```python
from build123d import *

# Parameters (mm, degrees)
SKETCH1_W           = 249.00380235
SKETCH1_H           = 131.677440474
BOSS_EXTRUDE1_DEPTH = 192
CHAMFER1_SIZE       = 100
SKETCH2_W           = 249.00380235
SKETCH2_H           = 141.421356237
SKETCH2_W_2         = 215.26057226
SKETCH2_H_2         = 100.329330499
BOSS_EXTRUDE2_DEPTH = 10
SHELL1_START        = -114.501901175
SHELL1_DEPTH        = 229.00380235
BOSS_EXTRUDE3_DEPTH = 5
SKETCH4_W           = 5
SKETCH4_H           = 182
BOSS_EXTRUDE4_DEPTH = 5


# Read off the part's stored shape, not the designer's step: Shell1
with BuildPart() as part:
    # Sketch1 → Boss-Extrude1 (new body)
    with BuildSketch(Plane(origin=(0, 0, 0), x_dir=(1, 0, 0), z_dir=(0, 1, 0))):
        Rectangle(SKETCH1_W, SKETCH1_H)
    extrude(amount=BOSS_EXTRUDE1_DEPTH)

    # Chamfer1
    chamfer1_edges = [part.edges().sort_by_distance(p)[0] for p in [
        (0, 192, 65.838720237),
    ]]
    chamfer(chamfer1_edges, length=CHAMFER1_SIZE)

    # Sketch2 → Boss-Extrude2 (add)
    with BuildSketch(Plane(origin=(0, 78.919360119, 78.919360119), x_dir=(1, 0, 0), z_dir=(0, 0.7071067811865464, 0.7071067811865487))):
        with Locations((0, 89.209496444)):
            Rectangle(SKETCH2_W, SKETCH2_H)
        with Locations((0, 89.209496444)):
            Rectangle(SKETCH2_W_2, SKETCH2_H_2, mode=Mode.SUBTRACT)
    extrude(amount=BOSS_EXTRUDE2_DEPTH)

    # Shell1 outline → Shell1 (cut)
    with BuildSketch(Plane.YZ.offset(SHELL1_START)):
        Polygon((96.142135624, 55.838720237), (10, 55.838720237), (10, -65.838720237), (182, -65.838720237), (182, -30.019144139), (184.928932188, -27.090211951), (99.071067812, 58.767652425), align=None)
    extrude(amount=SHELL1_DEPTH, mode=Mode.SUBTRACT)

    # Sketch3 → Boss-Extrude3 (add)
    with BuildSketch(Plane(origin=(0, 0, -65.838720237), x_dir=(-1, 0, 0), z_dir=(0, 0, -1))):
        Polygon((-114.501901175, 10), (-114.501901175, 182), (-114.501901175, 192), (-124.501901175, 192), (-124.501901175, 0), (124.501901175, 0), (124.501901175, 192), (114.501901175, 192), (114.501901175, 182), (114.501901175, 10), align=None)
    extrude(amount=BOSS_EXTRUDE3_DEPTH)

    # Sketch4 → Boss-Extrude4 (add)
    with BuildSketch(Plane(origin=(0, 0, -70.838720237), x_dir=(-1, 0, 0), z_dir=(0, 0, -1))):
        Polygon((124.501901175, 192), (114.501901175, 192), (114.501901175, 10), (-114.501901175, 10), (-114.501901175, 192), (-124.501901175, 192), (-124.501901175, 0), (124.501901175, 0), align=None)
        with Locations((112.001901175, 101)):
            Rectangle(SKETCH4_W, SKETCH4_H)
        with Locations((-112.001901175, 101)):
            Rectangle(SKETCH4_W, SKETCH4_H)
    extrude(amount=BOSS_EXTRUDE4_DEPTH)


solid = part.part
```
Geometry: final body of the model. Coordinates: model frame, mm. A direction names the side the tool comes from. Round coordinates to 2 decimals unless told otherwise and drop trailing zeros. Write each loop counter-clockwise with the first axis right and the second up, starting at its lowest first coordinate (ties: lowest second). Pieces come first, ordered by that corner, then holes. Notation, with made-up numbers: (66.5, -17.75) -> (91.5, -17.75) arc R24 ccw to (91.5, 6.25) -> close; hole circle Ø8 at (45.5, 6.25). An arc over 180 degrees is marked (long way). Use CSV: the item, a comma, the result in double quotes. Start each with the question number.
Q1. Section D-D (z = 23). Return loops of the section in (x, y), plus the area to 3 significant figures.
Q2. Line query: L1, parallel to Y at x = -92, z = -65; L2, parallel to X at y = 25.5, z = -51; L3, parallel to Z at x = -114, y = 91. Output: solid intervals per line, ascending.
Q3. Section B-B (x = 27). Return loops of the section in (y, z).
Q4. First-contact query: pin 1 Ø2.5 at (x, y) = (-112, 128) entering from +Z; pin 2 Ø8 at (x, z) = (13, -18) entering from +Y; pin 3 Ø5.5 at (x, y) = (111, 82) entering from +Z; pin 4 Ø18 at (x, z) = (25.5, -43) entering from -Y. Flat tips, straight axial feed; report the tip coordinate or a pass-through.
Q5. Section A-A (y = 15). Return loops of the section in (x, z).
Q6. Section C-C (y = 160). Return loops of the section in (x, z), plus the area to 3 significant figures.
Q7. Reachability of faces 5 (the face through (-2, 192, -50)), 6 (the face through (-114.502, 82, -5)), 7 (the face through (-1.507, 110.014, 54.797)), 8 (the face through (-1.743, 95.486, 69.325)), 9 (the face through (-1.507, 180.958, -16.147)) from +Z, -Z, +X, -X, +Y, -Y: full face, straight path, thin tool, end or side. Return the list, or none.
Q8. Pull-direction query (X, two-part tool) for faces 1 (the face through (-2, 54, 55.839)), 2 (the face through (-124.502, 76, 0)), 3 (the face through (124.502, 79, -17)), 4 (the face through (-2, 45, 65.839)); classes: pulls with the +X half, pulls with the -X half, needs draft (parallel to the pull), parting line crosses it, or undercut.
Result sheet:
1,outline,"(-124.5, 0) -> (124.5, 0) -> (124.5, 148.98) -> (107.63, 148.98) -> (107.63, 134.84) -> (114.5, 134.84) -> (114.5, 10) -> (-114.5, 10) -> (-114.5, 134.84) -> (-107.63, 134.84) -> (-107.63, 148.98) -> (-124.5, 148.98) -> close"
1,area,"5,460 mm²"
2,L1,"0 to 10, 182 to 192"
2,L2,"-124.5 to -114.5, 114.5 to 124.5"
2,L3,"-75.84 to -70.84, 55.84 to 65.84"
3,outline,"(0, -75.84) -> (10, -75.84) -> (10, 55.84) -> (96.14, 55.84) -> (99.07, 58.77) -> (106.53, 51.31) -> (113.6, 58.38) -> (99.07, 72.91) -> (92, 65.84) -> (0, 65.84) -> close; (177.47, -19.63) -> (184.93, -27.09) -> (182, -30.02) -> (182, -65.84) -> (192, -65.84) -> (192, -34.16) -> (199.07, -27.09) -> (184.54, -12.56) -> close"
4,pin 1,"z = 45.23"
4,pin 2,"y = 193.98"
4,pin 3,"z = 65.84"
4,pin 4,"y = 0"
5,outline,"(-124.5, -75.84) -> (-109.5, -75.84) -> (-109.5, -70.84) -> (-114.5, -70.84) -> (-114.5, 55.84) -> (114.5, 55.84) -> (114.5, -70.84) -> (109.5, -70.84) -> (109.5, -75.84) -> (124.5, -75.84) -> (124.5, 65.84) -> (-124.5, 65.84) -> close"
6,outline,"(-124.5, -75.84) -> (-109.5, -75.84) -> (-109.5, -70.84) -> (-114.5, -70.84) -> (-114.5, -2.16) -> (-107.63, -2.16) -> (-107.63, 11.98) -> (-124.5, 11.98) -> close; (107.63, -2.16) -> (114.5, -2.16) -> (114.5, -70.84) -> (109.5, -70.84) -> (109.5, -75.84) -> (124.5, -75.84) -> (124.5, 11.98) -> (107.63, 11.98) -> close"
6,area,"2,000 mm²"
7,face 5,"-Z, +X, -X, +Y"
7,face 6,"none"
7,face 7,"-Z, +Y"
7,face 8,"+Z, +X, -X, -Y"
7,face 9,"+Z"
8,face 1,"undercut"
8,face 2,"pulls with the -X half"
8,face 3,"pulls with the +X half"
8,face 4,"needs draft"
